```python
from build123d import *

# Parameters (mm, degrees)
SKETCH_1_W          = 44
SKETCH_1_H          = 42
EXTRUDE_1_DEPTH     = 9.5
SKETCH_2_R          = 11.5
CUT_EXTRUDE_1_DEPTH = 62.565006294
FILLET_1_R          = 3
SKETCH_5_R          = 1.6
CUT_EXTRUDE_2_DEPTH = 62.565006294
SKETCH_8_W          = 3.85
SKETCH_8_H          = 9.5
CUT_EXTRUDE_3_DEPTH = 1.5


with BuildPart() as part:
    # 草图1 → 凸台-拉伸1 (new body)
    with BuildSketch(Plane(origin=(0, 0, 0), x_dir=(1, 0, 0), z_dir=(0, 1, 0))):
        with Locations((22, -21)):
            Rectangle(SKETCH_1_W, SKETCH_1_H)
    extrude(amount=EXTRUDE_1_DEPTH)

    # 草图2 → 切除-拉伸1 (cut, through all)
    with BuildSketch(Plane(origin=(0, 9.5, 0), x_dir=(1, 0, 0), z_dir=(0, 1, 0))):
        with Locations(Location((21.15, -20.85, 0), (0, 0, 270))):
            Circle(SKETCH_2_R)
    extrude(amount=-CUT_EXTRUDE_1_DEPTH, mode=Mode.SUBTRACT)

    # 圆角1
    fillet_1_edges = [part.edges().sort_by_distance(p)[0] for p in [
        (0, 4.75, 0),
        (44, 4.75, 0),
        (44, 4.75, 42),
        (0, 4.75, 42),
    ]]
    fillet(fillet_1_edges, radius=FILLET_1_R)

    # 草图5 → 切除-拉伸2 (cut, through all)
    with BuildSketch(Plane.XZ):
        with Locations(Location((36.65, 36.35, 0), (0, 0, 270))):
            Circle(SKETCH_5_R)
        with Locations(Location((5.65, 36.35, 0), (0, 0, 270))):
            Circle(SKETCH_5_R)
        with Locations(Location((5.65, 5.35, 0), (0, 0, 270))):
            Circle(SKETCH_5_R)
        with Locations(Location((36.65, 5.35, 0), (0, 0, 270))):
            Circle(SKETCH_5_R)
    extrude(amount=-CUT_EXTRUDE_2_DEPTH, mode=Mode.SUBTRACT)

    # 草图8 → 切除-拉伸3 (cut)
    with BuildSketch(Plane.ZY):
        with Locations((12, 4.75)):
            Rectangle(SKETCH_8_W, SKETCH_8_H)
        with Locations((30, 4.75)):
            Rectangle(SKETCH_8_W, SKETCH_8_H)
    extrude(amount=-CUT_EXTRUDE_3_DEPTH, mode=Mode.SUBTRACT)


solid = part.part
```
Build history of the part. All positions in model axes, mm. A direction names the side the tool comes from. Give positions to 0.01 mm unless a question says otherwise; leave off trailing zeros. Loops run counter-clockwise (first coordinate to the right, second up) from the corner with the lowest first, then second, coordinate; pieces in that order, holes last.
1) Band-saw the part on B-B on y = 1.25. List the corners of the cut face in (x, z) (3 decimals).
Values follow:
outline: (0, 3) arc R3 ccw to (3, 0) - (41, 0) arc R3 ccw to (44, 3) - (44, 39) arc R3 ccw to (41, 42) - (3, 42) arc R3 ccw to (0, 39) - (0, 31.925) - (1.5, 31.925) - (1.5, 28.075) - (0, 28.075) - (0, 13.925) - (1.5, 13.925) - (1.5, 10.075) - (0, 10.075) - close; hole circle Ø3.2 at (5.65, 5.35); hole circle Ø3.2 at (5.65, 36.35); hole circle Ø23 at (21.15, 20.85); hole circle Ø3.2 at (36.65, 5.35); hole circle Ø3.2 at (36.65, 36.35)
2) Probe line 1 along X through (y, z) = (4.5, 5.35); line 2 along Z through (x, y) = (36, 8.25); line 3 along X through (y, z) = (0.5, 21). List the from-to ranges inside material, lowest first.
Values follow:
line 1: x = 0 to 4.05, 7.25 to 35.05, 38.25 to 44
line 2: z = 0 to 3.89, 6.81 to 34.89, 37.81 to 42
line 3: x = 0 to 9.65, 32.65 to 44
3) Band-saw the part on A-A on x = 5.65. List the corners of the cut face in (y, z).
Values follow:
outline: (0, 0) - (9.5, 0) - (9.5, 3.75) - (0, 3.75) - close; (0, 6.95) - (9.5, 6.95) - (9.5, 34.75) - (0, 34.75) - close; (0, 37.95) - (9.5, 37.95) - (9.5, 42) - (0, 42) - close
4) Two-plate mould, pull along Z, no slides. Class faces 3 (the face through (22, 5, 0)), 4 (the face through (0.86, 4.82, 41.1)), 5 (the face through (35.68, 4.68, 37.62)): released by +Z, released by -Z, zero draft, split by the parting line, or undercut.
Values follow:
face 3: released by -Z
face 4: released by +Z
face 5: undercut
5) Band-saw the part on D-D on z = 19. List the corners of the cut face in (x, y), then the cut area to 3 significant figures.
Values follow:
outline: (0, 0) - (9.8, 0) - (9.8, 9.5) - (0, 9.5) - close; (32.5, 0) - (44, 0) - (44, 9.5) - (32.5, 9.5) - close
area: 202 mm2
6) 3-axis set-ups, long thin cutter, end or side, ignore diameter. For faces 1 (the face through (22, 5, 42)), 2 (the face through (1.5, 5, 30)): which of +Z, -Z, +X, -X, +Y, -Y reach the whole face in a straight line?
Values follow:
face 1: +Z, +X, -X, +Y, -Y
face 2: -X, +Y, -Y
7) Drop flat-ended pins along their axis: P1, Ø1.2, axis at y = 7, z = 13, coming from the -X side; P2, Ø1.6, axis at x = 1, y = 4.5, coming from the +Z side; P3, Ø1.2, axis at x = 1, y = 2.5, coming from the -Z side; P4, Ø2.5, axis at x = 5.65, z = 36.35, coming from the +Y side. Give the stop position or say it passes through.
Values follow:
P1: stops at x = 1.5
P2: stops at z = 41.75
P3: stops at z = 0.35
P4: passes through
8) Band-saw the part on C-C on z = 5.35. List the corners of the cut face in (x, y).
Values follow:
outline: (0, 0) - (4.05, 0) - (4.05, 9.5) - (0, 9.5) - close; (7.25, 0) - (35.05, 0) - (35.05, 9.5) - (7.25, 9.5) - close; (38.25, 0) - (44, 0) - (44, 9.5) - (38.25, 9.5) - close
